from build123d import *

# Parameters (mm, degrees)
BOSS_EXTRUDE1_DEPTH = 6.35
CUT_EXTRUDE1_REACH  = 8.35
SKETCH3_W           = 6.35
SKETCH3_H           = 12
CUT_EXTRUDE2_REACH  = 8.35
SKETCH5_R           = 1.6
CUT_EXTRUDE3_DEPTH  = 7.35
FILLET1_R           = 5


with BuildPart() as part:
    # Sketch1 → Boss-Extrude1 (new body)
    with BuildSketch(Plane(origin=(0, 0, 0), x_dir=(1, 0, 0), z_dir=(0, 1, 0))):
        with BuildLine():
            Line((-30, -122.105), (30, -122.105))
            Line((30, -122.105), (60, -139.425508076))
            Line((60, -139.425508076), (75, -113.444745962))
            Line((75, -113.444745962), (30, -87.463983849))
            Line((30, -87.463983849), (30, 0))
            ThreePointArc((30, 0), (0, 30), (-30, 0))
            Line((-30, 0), (-30, -87.463983849))
            Line((-30, -87.463983849), (-75, -113.444745962))
            Line((-75, -113.444745962), (-60, -139.425508076))
            Line((-60, -139.425508076), (-30, -122.105))
        make_face()
    extrude(amount=BOSS_EXTRUDE1_DEPTH)

    # Sketch3 → Cut-Extrude1 (cut, up to next)
    with BuildSketch(Plane(origin=(0, 6.35, 0), x_dir=(1, 0, 0), z_dir=(0, 1, 0)), mode=Mode.PRIVATE) as cut_extrude1_sk1:
        with Locations((-26.825, -104.105)):
            Rectangle(SKETCH3_W, SKETCH3_H)
    cut_extrude1_tool1 = extrude(cut_extrude1_sk1.sketch, amount=-CUT_EXTRUDE1_REACH, mode=Mode.PRIVATE) & part.part
    add(cut_extrude1_tool1.solids().sort_by_distance((-26.825, 6.35, 104.105))[0], mode=Mode.SUBTRACT)
    # Sketch3 → Cut-Extrude1 (cut, up to next)
    with BuildSketch(Plane(origin=(0, 6.35, 0), x_dir=(1, 0, 0), z_dir=(0, 1, 0)), mode=Mode.PRIVATE) as cut_extrude1_sk2:
        with Locations((-26.825, -80.105)):
            Rectangle(SKETCH3_W, SKETCH3_H)
    cut_extrude1_tool2 = extrude(cut_extrude1_sk2.sketch, amount=-CUT_EXTRUDE1_REACH, mode=Mode.PRIVATE) & part.part
    add(cut_extrude1_tool2.solids().sort_by_distance((-26.825, 6.35, 80.105))[0], mode=Mode.SUBTRACT)
    # Sketch3 → Cut-Extrude1 (cut, up to next)
    with BuildSketch(Plane(origin=(0, 6.35, 0), x_dir=(1, 0, 0), z_dir=(0, 1, 0)), mode=Mode.PRIVATE) as cut_extrude1_sk3:
        with Locations((-26.825, -56.105)):
            Rectangle(SKETCH3_W, SKETCH3_H)
    cut_extrude1_tool3 = extrude(cut_extrude1_sk3.sketch, amount=-CUT_EXTRUDE1_REACH, mode=Mode.PRIVATE) & part.part
    add(cut_extrude1_tool3.solids().sort_by_distance((-26.825, 6.35, 56.105))[0], mode=Mode.SUBTRACT)
    # Sketch3 → Cut-Extrude1 (cut, up to next)
    with BuildSketch(Plane(origin=(0, 6.35, 0), x_dir=(1, 0, 0), z_dir=(0, 1, 0)), mode=Mode.PRIVATE) as cut_extrude1_sk4:
        with Locations((-26.825, -32.105)):
            Rectangle(SKETCH3_W, SKETCH3_H)
    cut_extrude1_tool4 = extrude(cut_extrude1_sk4.sketch, amount=-CUT_EXTRUDE1_REACH, mode=Mode.PRIVATE) & part.part
    add(cut_extrude1_tool4.solids().sort_by_distance((-26.825, 6.35, 32.105))[0], mode=Mode.SUBTRACT)
    # Sketch3 → Cut-Extrude1 (cut, up to next)
    with BuildSketch(Plane(origin=(0, 6.35, 0), x_dir=(1, 0, 0), z_dir=(0, 1, 0)), mode=Mode.PRIVATE) as cut_extrude1_sk5:
        with Locations((26.825, -32.105)):
            Rectangle(SKETCH3_W, SKETCH3_H)
    cut_extrude1_tool5 = extrude(cut_extrude1_sk5.sketch, amount=-CUT_EXTRUDE1_REACH, mode=Mode.PRIVATE) & part.part
    add(cut_extrude1_tool5.solids().sort_by_distance((26.825, 6.35, 32.105))[0], mode=Mode.SUBTRACT)
    # Sketch3 → Cut-Extrude1 (cut, up to next)
    with BuildSketch(Plane(origin=(0, 6.35, 0), x_dir=(1, 0, 0), z_dir=(0, 1, 0)), mode=Mode.PRIVATE) as cut_extrude1_sk6:
        with Locations((26.825, -56.105)):
            Rectangle(SKETCH3_W, SKETCH3_H)
    cut_extrude1_tool6 = extrude(cut_extrude1_sk6.sketch, amount=-CUT_EXTRUDE1_REACH, mode=Mode.PRIVATE) & part.part
    add(cut_extrude1_tool6.solids().sort_by_distance((26.825, 6.35, 56.105))[0], mode=Mode.SUBTRACT)
    # Sketch3 → Cut-Extrude1 (cut, up to next)
    with BuildSketch(Plane(origin=(0, 6.35, 0), x_dir=(1, 0, 0), z_dir=(0, 1, 0)), mode=Mode.PRIVATE) as cut_extrude1_sk7:
        with Locations((26.825, -80.105)):
            Rectangle(SKETCH3_W, SKETCH3_H)
    cut_extrude1_tool7 = extrude(cut_extrude1_sk7.sketch, amount=-CUT_EXTRUDE1_REACH, mode=Mode.PRIVATE) & part.part
    add(cut_extrude1_tool7.solids().sort_by_distance((26.825, 6.35, 80.105))[0], mode=Mode.SUBTRACT)
    # Sketch3 → Cut-Extrude1 (cut, up to next)
    with BuildSketch(Plane(origin=(0, 6.35, 0), x_dir=(1, 0, 0), z_dir=(0, 1, 0)), mode=Mode.PRIVATE) as cut_extrude1_sk8:
        with Locations((26.825, -104.105)):
            Rectangle(SKETCH3_W, SKETCH3_H)
    cut_extrude1_tool8 = extrude(cut_extrude1_sk8.sketch, amount=-CUT_EXTRUDE1_REACH, mode=Mode.PRIVATE) & part.part
    add(cut_extrude1_tool8.solids().sort_by_distance((26.825, 6.35, 104.105))[0], mode=Mode.SUBTRACT)

    # Sketch4 → Cut-Extrude2 (cut, up to next)
    with BuildSketch(Plane(origin=(0, 6.35, 0), x_dir=(1, 0, 0), z_dir=(0, 1, 0)), mode=Mode.PRIVATE) as cut_extrude2_sk1:
        Polygon((23.65, -30.505), (22.15, -30.505), (22.15, -29.305), (19.65, -29.305), (19.65, -30.505), (14.65, -30.505), (14.65, -33.705), (19.65, -33.705), (19.65, -34.905), (22.15, -34.905), (22.15, -33.705), (23.65, -33.705), align=None)
    cut_extrude2_tool1 = extrude(cut_extrude2_sk1.sketch, amount=-CUT_EXTRUDE2_REACH, mode=Mode.PRIVATE) & part.part
    add(cut_extrude2_tool1.solids().sort_by_distance((19.451724, 6.35, 32.105))[0], mode=Mode.SUBTRACT)
    # Sketch4 → Cut-Extrude2 (cut, up to next)
    with BuildSketch(Plane(origin=(0, 6.35, 0), x_dir=(1, 0, 0), z_dir=(0, 1, 0)), mode=Mode.PRIVATE) as cut_extrude2_sk2:
        Polygon((22.15, -53.305), (19.65, -53.305), (19.65, -54.505), (14.65, -54.505), (14.65, -57.705), (19.65, -57.705), (19.65, -58.905), (22.15, -58.905), (22.15, -57.705), (23.65, -57.705), (23.65, -54.505), (22.15, -54.505), align=None)
    cut_extrude2_tool2 = extrude(cut_extrude2_sk2.sketch, amount=-CUT_EXTRUDE2_REACH, mode=Mode.PRIVATE) & part.part
    add(cut_extrude2_tool2.solids().sort_by_distance((19.451724, 6.35, 56.105))[0], mode=Mode.SUBTRACT)
    # Sketch4 → Cut-Extrude2 (cut, up to next)
    with BuildSketch(Plane(origin=(0, 6.35, 0), x_dir=(1, 0, 0), z_dir=(0, 1, 0)), mode=Mode.PRIVATE) as cut_extrude2_sk3:
        Polygon((22.15, -77.305), (19.65, -77.305), (19.65, -78.505), (14.65, -78.505), (14.65, -81.705), (19.65, -81.705), (19.65, -82.905), (22.15, -82.905), (22.15, -81.705), (23.65, -81.705), (23.65, -78.505), (22.15, -78.505), align=None)
    cut_extrude2_tool3 = extrude(cut_extrude2_sk3.sketch, amount=-CUT_EXTRUDE2_REACH, mode=Mode.PRIVATE) & part.part
    add(cut_extrude2_tool3.solids().sort_by_distance((19.451724, 6.35, 80.105))[0], mode=Mode.SUBTRACT)
    # Sketch4 → Cut-Extrude2 (cut, up to next)
    with BuildSketch(Plane(origin=(0, 6.35, 0), x_dir=(1, 0, 0), z_dir=(0, 1, 0)), mode=Mode.PRIVATE) as cut_extrude2_sk4:
        Polygon((-22.15, -78.505), (-22.15, -77.305), (-19.65, -77.305), (-19.65, -78.505), (-14.65, -78.505), (-14.65, -81.705), (-19.65, -81.705), (-19.65, -82.905), (-22.15, -82.905), (-22.15, -81.705), (-23.65, -81.705), (-23.65, -78.505), align=None)
    cut_extrude2_tool4 = extrude(cut_extrude2_sk4.sketch, amount=-CUT_EXTRUDE2_REACH, mode=Mode.PRIVATE) & part.part
    add(cut_extrude2_tool4.solids().sort_by_distance((-19.451724, 6.35, 80.105))[0], mode=Mode.SUBTRACT)
    # Sketch4 → Cut-Extrude2 (cut, up to next)
    with BuildSketch(Plane(origin=(0, 6.35, 0), x_dir=(1, 0, 0), z_dir=(0, 1, 0)), mode=Mode.PRIVATE) as cut_extrude2_sk5:
        Polygon((-22.15, -54.505), (-22.15, -53.305), (-19.65, -53.305), (-19.65, -54.505), (-14.65, -54.505), (-14.65, -57.705), (-19.65, -57.705), (-19.65, -58.905), (-22.15, -58.905), (-22.15, -57.705), (-23.65, -57.705), (-23.65, -54.505), align=None)
    cut_extrude2_tool5 = extrude(cut_extrude2_sk5.sketch, amount=-CUT_EXTRUDE2_REACH, mode=Mode.PRIVATE) & part.part
    add(cut_extrude2_tool5.solids().sort_by_distance((-19.451724, 6.35, 56.105))[0], mode=Mode.SUBTRACT)
    # Sketch4 → Cut-Extrude2 (cut, up to next)
    with BuildSketch(Plane(origin=(0, 6.35, 0), x_dir=(1, 0, 0), z_dir=(0, 1, 0)), mode=Mode.PRIVATE) as cut_extrude2_sk6:
        Polygon((-19.65, -33.705), (-14.65, -33.705), (-14.65, -30.505), (-19.65, -30.505), (-19.65, -29.305), (-22.15, -29.305), (-22.15, -30.505), (-23.65, -30.505), (-23.65, -33.705), (-22.15, -33.705), (-22.15, -34.905), (-19.65, -34.905), align=None)
    cut_extrude2_tool6 = extrude(cut_extrude2_sk6.sketch, amount=-CUT_EXTRUDE2_REACH, mode=Mode.PRIVATE) & part.part
    add(cut_extrude2_tool6.solids().sort_by_distance((-19.451724, 6.35, 32.105))[0], mode=Mode.SUBTRACT)

    # Sketch5 → Cut-Extrude3 (cut, through all)
    with BuildSketch(Plane(origin=(0, 6.35, 0), x_dir=(1, 0, 0), z_dir=(0, 1, 0))):
        with Locations((-17.033871657, 20.300177743)):
            Circle(SKETCH5_R)
        with Locations((17.033871657, 20.300177743)):
            Circle(SKETCH5_R)
    extrude(amount=-CUT_EXTRUDE3_DEPTH, mode=Mode.SUBTRACT)

    # Fillet1
    fillet1_edges = [part.edges().sort_by_distance(p)[0] for p in [
        (75, 3.175, 113.444745962),
        (60, 3.175, 139.425508076),
        (30, 3.175, 122.105),
        (-30, 3.175, 122.105),
        (-60, 3.175, 139.425508076),
        (-75, 3.175, 113.444745962),
    ]]
    fillet(fillet1_edges, radius=FILLET1_R)


solid = part.part
Source: CAD feature listing. Evaluate the final solid. Frame: model axes, mm. A direction names the side the tool comes from. Coordinates: 2 decimals unless noted, no trailing zeros. Loops run counter-clockwise (first coordinate to the right, second up) from the corner with the lowest first, then second, coordinate; pieces in that order, holes last. Notation, with made-up numbers: M 18,-18 L 57,-18 A27 ccw 57,16 Z; hole C -33.75,-22 d2. An arc over 180 degrees is marked long. Answer in a Markdown table with one row per item.
Q1. Draft query along X for faces 6 (the flat face through (-27, 3, 110.105)), 7 (the flat face through (27, 3, 62.105)), 8 (the flat face through (23.65, 3, 28)). Return one class per face: pulls with the +X half, pulls with the -X half, needs draft (parallel to the pull), parting line crosses it, or undercut.
Answers below:
| item | result |
|---|---|
| face 6 | undercut |
| face 7 | needs draft |
| face 8 | pulls with the +X half |
Q2. Section D-D on z = 18.5. Return the cut outline in (x, y).
Answers below:
| item | result |
|---|---|
| outline | M -30,0 L 30,0 L 30,6.35 L -30,6.35 Z |
Q3. First-contact query: pin 1 (1.2 mm diameter, centred on x = 23, y = 3, fed in from +Z) (3 decimals); pin 2 (8 mm diameter, centred on x = 1.5, z = 19, fed in from -Y); pin 3 (2 mm diameter, centred on y = 4.5, z = 27.5, fed in from +X); pin 4 (2 mm diameter, centred on x = -20.5, y = 4.5, fed in from -Z). Flat tips, straight axial feed; report the tip coordinate or a pass-through.
Answers below:
| item | result |
|---|---|
| pin 1 | stops at z = 122.105 |
| pin 2 | stops at y = 0 |
| pin 3 | stops at x = 23.65 |
| pin 4 | stops at z = -22.8 |
Q4. Section C-C on y = 4. State how many separate pieces and enclosed holes the cut face has, plus the area to 3 significant figures.
Answers below:
| item | result |
|---|---|
| separate pieces | 1 |
| enclosed holes | 4 |
| area | 10,500 mm^2 |
Q5. Section B-B on x = 0. Return the cut outline in (y, z) (3 decimals), plus the area to 3 significant figures.
Answers below:
| item | result |
|---|---|
| outline | M 0,-30 L 6.35,-30 L 6.35,122.105 L 0,122.105 Z |
| area | 966 mm^2 |
Q6. Section A-A on z = 104.5. Return the cut outline in (x, y).
Answers below:
| item | result |
|---|---|
| outline | M -59.51,0 L -30,0 L -30,6.35 L -59.51,6.35 Z; M -23.65,0 L 23.65,0 L 23.65,6.35 L -23.65,6.35 Z; M 30,0 L 59.51,0 L 59.51,6.35 L 30,6.35 Z |
Q7. Set-up query: faces 1 (the flat face through (43.24, 3.13, 129.75)), 2 (the flat face through (27, 3, 26.105)), 3 (the flat face through (-30, 3, 44)), 4 (the flat face through (-27, 3, 74.105)), 5 (the flat face through (23.65, 3, 104)). Return all of +Z, -Z, +X, -X, +Y, -Y with unobstructed straight access to the full face (end or side cutting, diameter ignored); none if empty.
Answers below:
| item | result |
|---|---|
| face 1 | +Z, +Y, -Y |
| face 2 | +X, +Y, -Y |
| face 3 | -Z, -X, +Y, -Y |
| face 4 | -X, +Y, -Y |
| face 5 | +Y, -Y |
Q8. Ray query, probe 1 along X at (y, z) = (0.75, -19); probe 2 along Z at (x, y) = (23, 4.25) (3 decimals); probe 3 along Z at (x, y) = (20, 1) (3 decimals). Return the intervals inside material, ascending. Write a range as from..to.
Answers below:
| item | result |
|---|---|
| probe 1 | x = -23.22..-17.97, -16.1..16.1, 17.97..23.22 |
| probe 2 | z = -19.261..30.505, 33.705..54.505, 57.705..78.505, 81.705..122.105 |
| probe 3 | z = -22.361..29.305, 34.905..53.305, 58.905..77.305, 82.905..122.105 |
